from build123d import *

# Parameters (mm, degrees)
F0_W     = 1854.2
F0_H     = 38.1
F0_W_2   = 38.1
F0_H_2   = 298.45
F0_H_3   = 336.55
F0_H_4   = 679.45
F1_DEPTH = 101.6


with BuildPart() as f1:
    # F0 (on Top) → F1 (new body)
    with BuildSketch(Plane.XY):
        with Locations((965.2, 2012.95)):
            Rectangle(F0_W, F0_H)
        Polygon((1892.3, 1955.8), (1892.3, 1993.9), (38.1, 1993.9), (38.1, 1955.8), (362.600505, 1955.8), (400.700505, 1955.8), (945.00792, 1955.8), (983.10792, 1955.8), (1531.078815, 1955.8), (1569.178815, 1955.8), align=None)
        Polygon((0, 0), (38.1, 0), (38.1, 38.1), (38.1, 76.2), (38.1, 755.65), (38.1, 793.75), (38.1, 831.85), (38.1, 1168.4), (38.1, 1206.5), (38.1, 1244.6), (38.1, 1581.15), (38.1, 1619.25), (38.1, 1657.35), (38.1, 1955.8), (38.1, 1993.9), (38.1, 2032), (0, 2032), align=None)
        with Locations((381.650505, 1806.575)):
            Rectangle(F0_W_2, F0_H_2)
        Polygon((1892.3, 1619.25), (1892.3, 1657.35), (1569.178815, 1657.35), (1531.078815, 1657.35), (983.10792, 1657.35), (945.00792, 1657.35), (400.700505, 1657.35), (362.600505, 1657.35), (38.1, 1657.35), (38.1, 1619.25), align=None)
        with Locations((964.05792, 1806.575)):
            Rectangle(F0_W_2, F0_H_2)
        with Locations((1550.128815, 1806.575)):
            Rectangle(F0_W_2, F0_H_2)
        Polygon((1892.3, 38.1), (1892.3, 0), (1930.4, 0), (1930.4, 2032), (1892.3, 2032), (1892.3, 1993.9), (1892.3, 1955.8), (1892.3, 1657.35), (1892.3, 1619.25), (1892.3, 1581.15), (1892.3, 1244.6), (1892.3, 1206.5), (1892.3, 1168.4), (1892.3, 831.85), (1892.3, 793.75), (1892.3, 755.65), (1892.3, 76.2), align=None)
        with Locations((1257.2695, 1412.875)):
            Rectangle(F0_W_2, F0_H_3)
        with Locations((672.729013, 1412.875)):
            Rectangle(F0_W_2, F0_H_3)
        Polygon((38.1, 1206.5), (1892.3, 1206.5), (1892.3, 1244.6), (1276.3195, 1244.6), (1238.2195, 1244.6), (691.779013, 1244.6), (653.679013, 1244.6), (38.1, 1244.6), align=None)
        Polygon((1571.134563, 1168.4), (1892.3, 1168.4), (1892.3, 1206.5), (38.1, 1206.5), (38.1, 1168.4), (361.264458, 1168.4), (399.364458, 1168.4), (945.316911, 1168.4), (983.416911, 1168.4), (1533.034563, 1168.4), align=None)
        with Locations((380.314458, 1000.125)):
            Rectangle(F0_W_2, F0_H_3)
        with Locations((964.366911, 1000.125)):
            Rectangle(F0_W_2, F0_H_3)
        with Locations((1552.084563, 1000.125)):
            Rectangle(F0_W_2, F0_H_3)
        Polygon((1587.552901, 755.65), (1892.3, 755.65), (1892.3, 793.75), (38.1, 793.75), (38.1, 755.65), (342.952732, 755.65), (381.052732, 755.65), (419.152732, 755.65), (654.369056, 755.65), (692.469056, 755.65), (947.420001, 755.65), (985.520001, 755.65), (1238.64913, 755.65), (1276.74913, 755.65), (1511.352901, 755.65), (1549.452901, 755.65), align=None)
        with Locations((1568.502901, 415.925)):
            Rectangle(F0_W_2, F0_H_4)
        with Locations((1530.402901, 415.925)):
            Rectangle(F0_W_2, F0_H_4)
        with Locations((1257.69913, 415.925)):
            Rectangle(F0_W_2, F0_H_4)
        with Locations((966.470001, 415.925)):
            Rectangle(F0_W_2, F0_H_4)
        with Locations((673.419056, 415.925)):
            Rectangle(F0_W_2, F0_H_4)
        with Locations((400.102732, 415.925)):
            Rectangle(F0_W_2, F0_H_4)
        with Locations((362.002732, 415.925)):
            Rectangle(F0_W_2, F0_H_4)
        Polygon((38.1, 38.1), (1892.3, 38.1), (1892.3, 76.2), (1587.552901, 76.2), (1549.452901, 76.2), (1511.352901, 76.2), (1276.74913, 76.2), (1238.64913, 76.2), (985.520001, 76.2), (947.420001, 76.2), (692.469056, 76.2), (654.369056, 76.2), (419.152732, 76.2), (381.052732, 76.2), (342.952732, 76.2), (38.1, 76.2), align=None)
        with Locations((965.2, 19.05)):
            Rectangle(F0_W, F0_H)
        Polygon((38.1, 793.75), (1892.3, 793.75), (1892.3, 831.85), (1571.134563, 831.85), (1533.034563, 831.85), (983.416911, 831.85), (945.316911, 831.85), (399.364458, 831.85), (361.264458, 831.85), (38.1, 831.85), align=None)
        Polygon((1892.3, 1581.15), (1892.3, 1619.25), (38.1, 1619.25), (38.1, 1581.15), (653.679013, 1581.15), (691.779013, 1581.15), (1238.2195, 1581.15), (1276.3195, 1581.15), align=None)
    extrude(amount=-F1_DEPTH)


solid = f1.part
The listing builds one solid part. Answer for the finished solid, in the listing's coordinates (mm). Coordinates: 2 decimals unless noted, no trailing zeros. Loops run counter-clockwise (first coordinate to the right, second up) from the corner with the lowest first, then second, coordinate; pieces in that order, holes last. Notation, with made-up numbers: (-34.5, 18.25) -> (-17.5, 18.25) arc R15 cw to (-17.5, 36.25) -> close; hole circle Ø9 at (-2, -10.5). An arc over 180 degrees is marked (long way). Write item = value, one per line. Start each with the question number.
1) A cutting plane is placed at A-A (x = 738.5). Give the vertices of the cut face in (y, z).
2) Straight lines are drawn through the part: line 1 (Y direction, x = 1653, z = -13.5); line 2 (X direction, y = 1483, z = -75); line 3 (X direction, y = 1720.5, z = -44). For each, find the intervals that lie inside material, in ascending order. Write a range as from..to.
3) A cutting plane is placed at C-C (y = 277.5). Give the vertices of the cut face in (x, z).
4) The mould has two halves that part along Y. Classify faces 1 (the face through (979, 2032, -50)), 2 (the face through (1531.079, 1804, -50)), 3 (the face through (961, 1096, 0)): released by +Y, released by -Y, zero draft, split by the parting line, or undercut.
5) A cutting plane is placed at B-B (y = 1539). Give the vertices of the cut face in (x, z), then the cut area to 3 significant figures.
6) A cutting plane is placed at D-D (y = 1841). Give the vertices of the cut face in (x, z), then the cut area to 3 significant figures.
Responses:
q1.outline = (0, -101.6) -> (76.2, -101.6) -> (76.2, 0) -> (0, 0) -> close; (755.65, -101.6) -> (831.85, -101.6) -> (831.85, 0) -> (755.65, 0) -> close; (1168.4, -101.6) -> (1244.6, -101.6) -> (1244.6, 0) -> (1168.4, 0) -> close; (1581.15, -101.6) -> (1657.35, -101.6) -> (1657.35, 0) -> (1581.15, 0) -> close; (1955.8, -101.6) -> (2032, -101.6) -> (2032, 0) -> (1955.8, 0) -> close
q2.line_1 = 0..76.2, 755.65..831.85, 1168.4..1244.6, 1581.15..1657.35, 1955.8..2032
q2.line_2 = 0..38.1, 653.68..691.78, 1238.22..1276.32, 1892.3..1930.4
q2.line_3 = 0..38.1, 362.6..400.7, 945.01..983.11, 1531.08..1569.18, 1892.3..1930.4
q3.outline = (0, -101.6) -> (38.1, -101.6) -> (38.1, 0) -> (0, 0) -> close; (342.95, -101.6) -> (419.15, -101.6) -> (419.15, 0) -> (342.95, 0) -> close; (654.37, -101.6) -> (692.47, -101.6) -> (692.47, 0) -> (654.37, 0) -> close; (947.42, -101.6) -> (985.52, -101.6) -> (985.52, 0) -> (947.42, 0) -> close; (1238.65, -101.6) -> (1276.75, -101.6) -> (1276.75, 0) -> (1238.65, 0) -> close; (1511.35, -101.6) -> (1587.55, -101.6) -> (1587.55, 0) -> (1511.35, 0) -> close; (1892.3, -101.6) -> (1930.4, -101.6) -> (1930.4, 0) -> (1892.3, 0) -> close
q4.face_1 = released by +Y
q4.face_2 = undercut
q4.face_3 = zero draft
q5.outline = (0, -101.6) -> (38.1, -101.6) -> (38.1, 0) -> (0, 0) -> close; (653.68, -101.6) -> (691.78, -101.6) -> (691.78, 0) -> (653.68, 0) -> close; (1238.22, -101.6) -> (1276.32, -101.6) -> (1276.32, 0) -> (1238.22, 0) -> close; (1892.3, -101.6) -> (1930.4, -101.6) -> (1930.4, 0) -> (1892.3, 0) -> close
q5.area = 15,500 mm²
q6.outline = (0, -101.6) -> (38.1, -101.6) -> (38.1, 0) -> (0, 0) -> close; (362.6, -101.6) -> (400.7, -101.6) -> (400.7, 0) -> (362.6, 0) -> close; (945.01, -101.6) -> (983.11, -101.6) -> (983.11, 0) -> (945.01, 0) -> close; (1531.08, -101.6) -> (1569.18, -101.6) -> (1569.18, 0) -> (1531.08, 0) -> close; (1892.3, -101.6) -> (1930.4, -101.6) -> (1930.4, 0) -> (1892.3, 0) -> close
q6.area = 19,400 mm²
